```python
from build123d import *

# Parameters (mm, degrees)
SKETCH1_W                = 20
SKETCH1_H                = 6
BOSS_EXTRUDE1_DEPTH      = 14
CUT_EXTRUDE1_REACH       = 9.69
SKETCH2_R                = 2.6
SKETCH3_W                = 14
SKETCH3_H                = 20
BOSS_EXTRUDE2_DEPTH      = 3
BOSS_EXTRUDE2_DEPTH_BACK = 3
SKETCH4_R                = 1.025
CUT_EXTRUDE4_DEPTH       = 6
SKETCH5_W                = 5.5
SKETCH5_H                = 8
CUT_EXTRUDE5_DEPTH       = 6
CHAMFER1_SIZE            = 2
CHAMFER2_SIZE            = 2.5
SKETCH6_W                = 5.5
SKETCH6_H                = 0.407228715
CUT_EXTRUDE6_DEPTH       = 2.69
SKETCH7_W                = 2
SKETCH7_H                = 4.5
BOSS_EXTRUDE3_DEPTH      = 6


with BuildPart() as part:
    # Sketch1 → Boss-Extrude1 (new body)
    with BuildSketch(Plane(origin=(32.364284334, 0, 0), x_dir=(0, 0, -1), z_dir=(1, 0, 0))):
        with Locations((-7.875866483, 38.765059464)):
            Rectangle(SKETCH1_W, SKETCH1_H)
        with BuildLine():
            Line((-12.22448084, 35.533673821), (-10.765866483, 34.075059464))
            Line((-10.765866483, 34.075059464), (-4.985866483, 34.075059464))
            Line((-4.985866483, 34.075059464), (-3.527252126, 35.533673821))
            ThreePointArc((-3.527252126, 35.533673821), (-3.27095768, 35.704924294), (-2.968637768, 35.765059464))
            Line((-2.968637768, 35.765059464), (-12.783095197, 35.765059464))
            ThreePointArc((-12.783095197, 35.765059464), (-12.480775285, 35.704924294), (-12.22448084, 35.533673821))
        make_face()
    extrude(amount=BOSS_EXTRUDE1_DEPTH)

    # Sketch2 → Cut-Extrude1 (cut, up to next)
    with BuildSketch(Plane.XZ.offset(-34.075059464), mode=Mode.PRIVATE) as cut_extrude1_sk1:
        with Locations((37.864284334, 7.875866483)):
            Circle(SKETCH2_R)
    cut_extrude1_tool1 = extrude(cut_extrude1_sk1.sketch, amount=-CUT_EXTRUDE1_REACH, mode=Mode.PRIVATE) & part.part
    add(cut_extrude1_tool1.solids().sort_by_distance((37.864284, 34.075059, 7.875866))[0], mode=Mode.SUBTRACT)

    # Sketch3 → Boss-Extrude2 (add, two sides)
    with BuildSketch(Plane.XY.offset(17.875866483)) as boss_extrude2_sk:
        with Locations((39.364284334, 45.765059464)):
            Rectangle(SKETCH3_W, SKETCH3_H)
    extrude(amount=BOSS_EXTRUDE2_DEPTH)
    extrude(boss_extrude2_sk.sketch, amount=-BOSS_EXTRUDE2_DEPTH_BACK)

    # Sketch4 → Cut-Extrude4 (cut)
    with BuildSketch(Plane.XY.offset(20.875866483)):
        with Locations((39.364284334, 50.565059464)):
            Circle(SKETCH4_R)
        with Locations((39.364284334, 40.965059464)):
            Circle(SKETCH4_R)
    extrude(amount=-CUT_EXTRUDE4_DEPTH, mode=Mode.SUBTRACT)

    # Sketch5 → Cut-Extrude5 (cut)
    with BuildSketch(Plane(origin=(0, 41.765059464, 0), x_dir=(1, 0, 0), z_dir=(0, 1, 0))):
        with Locations((43.614284334, -1.875866483)):
            Rectangle(SKETCH5_W, SKETCH5_H)
    extrude(amount=-CUT_EXTRUDE5_DEPTH, mode=Mode.SUBTRACT)

    # Chamfer1
    chamfer1_edges = [part.edges().sort_by_distance(p)[0] for p in [
        (40.864284334, 38.765059464, 5.875866483),
    ]]
    chamfer(chamfer1_edges, length=CHAMFER1_SIZE)

    # Chamfer2
    chamfer2_edges = [part.edges().sort_by_distance(p)[0] for p in [
        (44.614284334, 35.765059464, 5.875866483),
    ]]
    chamfer(chamfer2_edges, length=CHAMFER2_SIZE)

    # Sketch6 → Cut-Extrude6 (cut, through all)
    with BuildSketch(Plane(origin=(0, 35.765059464, 0), x_dir=(1, 0, 0), z_dir=(0, 1, 0))):
        with Locations((43.614284334, -3.172252126)):
            Rectangle(SKETCH6_W, SKETCH6_H)
    extrude(amount=-CUT_EXTRUDE6_DEPTH, mode=Mode.SUBTRACT)

    # Sketch7 → Boss-Extrude3 (add)
    with BuildSketch(Plane.XY.offset(20.875866483)):
        Polygon((46.364284334, 55.765059464), (46.364284334, 65.765059464), (42.364284334, 65.765059464), (32.364284334, 55.765059464), align=None)
        with Locations((43.864284334, 61.015059464)):
            Rectangle(SKETCH7_W, SKETCH7_H, mode=Mode.SUBTRACT)
    extrude(amount=-BOSS_EXTRUDE3_DEPTH)


solid = part.part
```
For this review, take the finished solid that the model builds, in its own axes (mm). A direction names the side the tool comes from. Round coordinates to 2 decimals unless told otherwise and drop trailing zeros. Loops run counter-clockwise (first coordinate to the right, second up) from the corner with the lowest first, then second, coordinate; pieces in that order, holes last.
(1) Tool access review of faces 4 (the flat face through (39, 41, 14.876)), 5 (the flat face through (41, 51, 14.876)), 6 (the flat face through (44.864, 61, 18)), 7 (the flat face through (37, 35.765, 0)): name each direction out of +Z, -Z, +X, -X, +Y, -Y from which nothing blocks a thin tool from reaching the whole face with its end or side.
Returned:
face 4: +Z
face 5: -Z, +X, -X, +Y
face 6: +Z, -Z
face 7: -Z, +X, -X, -Y
(2) Clearance check with flat-ended pins moving along their axes: P1, Ø1, axis at x = 44.5, z = 18, coming from the -Y side; P2, Ø6, axis at x = 35, z = 11, coming from the +Y side; P3, Ø6, axis at x = 43.5, y = 52, coming from the -Z side. State where each tip first meets the part, or that it passes through.
Returned:
P1: stops at y = 35.77
P2: stops at y = 41.77
P3: stops at z = 14.88
(3) Mouldability with a two-part tool opening along X and no side actions: class faces 1 (the flat face through (32.364, 40, 12)), 2 (the flat face through (41, 41.765, 6)), 3 (the cylindrical face through (38.55, 40.34, 17.92)) as released by +X, released by -X, zero draft, split by the parting line, or undercut.
Returned:
face 1: released by -X
face 2: zero draft
face 3: undercut
(4) Wall thickness on line 1 along Y through (x, z) = (44.25, 19.5); line 2 along X through (y, z) = (37, 8); line 3 along Y through (x, z) = (38.75, 16.75): over which ranges is each line inside the solid? List them lowest first.
Returned:
line 1: y = 35.77 to 58.77, 63.27 to 65.77
line 2: x = 32.36 to 35.27, 40.46 to 46.36
line 3: y = 35.77 to 40.14, 41.79 to 49.74, 51.39 to 62.15
(5) We need section B-B (y = 40.5). Give the boundary of the cut face in (x, z), plus the area to 3 significant figures.
Returned:
outline: (32.36, -2.12) - (40.86, -2.12) - (40.86, 3.88) - (42.86, 5.88) - (46.36, 5.88) - (46.36, 20.88) - (40.28, 20.88) - (40.28, 14.88) - (38.45, 14.88) - (38.45, 20.88) - (32.36, 20.88) - close; hole circle Ø5.2 at (37.86, 7.88)
area: 248 mm2
(6) We need section D-D (y = 62.5). Give the boundary of the cut face in (x, z), plus the area to 3 significant figures.
Returned:
outline: (39.1, 14.88) - (42.86, 14.88) - (42.86, 20.88) - (39.1, 20.88) - close; (44.86, 14.88) - (46.36, 14.88) - (46.36, 20.88) - (44.86, 20.88) - close
area: 31.6 mm2
(7) We need section C-C (z = 6.75). Give the boundary of the cut face in (x, y), plus the area to 3 significant figures.
Returned:
outline: (32.36, 34.08) - (35.52, 34.08) - (35.52, 41.77) - (32.36, 41.77) - close; (40.21, 34.08) - (46.36, 34.08) - (46.36, 41.77) - (40.21, 41.77) - close
area: 71.6 mm2
(8) We need section A-A (x = 43.25). Give the boundary of the cut face in (y, z).
Returned:
outline: (34.08, 4.99) - (35.53, 3.53) arc R0.79 cw to (35.65, 3.38) - (35.77, 3.38) - (38.27, 5.88) - (41.77, 5.88) - (41.77, 14.88) - (58.77, 14.88) - (58.77, 20.88) - (35.77, 20.88) - (35.77, 12.78) arc R0.79 cw to (35.53, 12.22) - (34.08, 10.77) - close; (63.27, 14.88) - (65.77, 14.88) - (65.77, 20.88) - (63.27, 20.88) - close
